from build123d import *

# Parameters (mm, degrees)
SKETCH1_W           = 138
SKETCH1_H           = 108.5
SKETCH1_R           = 1.75
BOSS_EXTRUDE1_DEPTH = 10


with BuildPart() as part:
    # Sketch1 → Boss-Extrude1 (new body)
    with BuildSketch(Plane(origin=(0, 0, 0), x_dir=(1, 0, 0), z_dir=(0, 1, 0))):
        Rectangle(SKETCH1_W, SKETCH1_H)
        with Locations(Location((-64, 49, 0), (0, 0, 270))):  # turned: the seam where the file's is
            Circle(SKETCH1_R, mode=Mode.SUBTRACT)
        with Locations(Location((-64, -49, 0), (0, 0, 270))):  # turned: the seam where the file's is
            Circle(SKETCH1_R, mode=Mode.SUBTRACT)
        with Locations(Location((64, -49, 0), (0, 0, 270))):  # turned: the seam where the file's is
            Circle(SKETCH1_R, mode=Mode.SUBTRACT)
        with Locations(Location((64, 49, 0), (0, 0, 270))):  # turned: the seam where the file's is
            Circle(SKETCH1_R, mode=Mode.SUBTRACT)
        with Locations(Location((-57.5, 44, 0), (0, 0, 270))):  # turned: the seam where the file's is
            Circle(SKETCH1_R, mode=Mode.SUBTRACT)
        with Locations(Location((-17.5, 44, 0), (0, 0, 270))):  # turned: the seam where the file's is
            Circle(SKETCH1_R, mode=Mode.SUBTRACT)
        with Locations(Location((-17.5, -44, 0), (0, 0, 270))):  # turned: the seam where the file's is
            Circle(SKETCH1_R, mode=Mode.SUBTRACT)
        with Locations(Location((-57.5, -44, 0), (0, 0, 270))):  # turned: the seam where the file's is
            Circle(SKETCH1_R, mode=Mode.SUBTRACT)
        with Locations(Location((17.5, -44, 0), (0, 0, 270))):  # turned: the seam where the file's is
            Circle(SKETCH1_R, mode=Mode.SUBTRACT)
        with Locations(Location((57.5, -44, 0), (0, 0, 270))):  # turned: the seam where the file's is
            Circle(SKETCH1_R, mode=Mode.SUBTRACT)
        with Locations(Location((57.5, 44, 0), (0, 0, 270))):  # turned: the seam where the file's is
            Circle(SKETCH1_R, mode=Mode.SUBTRACT)
        with Locations(Location((17.5, 44, 0), (0, 0, 270))):  # turned: the seam where the file's is
            Circle(SKETCH1_R, mode=Mode.SUBTRACT)
    extrude(amount=BOSS_EXTRUDE1_DEPTH)


solid = part.part
The listing builds one solid part. Answer for the finished solid, in the listing's coordinates (mm). Give positions to 0.01 mm unless a question says otherwise; leave off trailing zeros. Write each loop counter-clockwise with the first axis right and the second up, starting at its lowest first coordinate (ties: lowest second). Pieces come first, ordered by that corner, then holes. Notation, with made-up numbers: (8.5, -33) -> (60.5, -33) arc R26 cw to (60.5, -3) -> close; hole circle Ø10 at (59.25, 62.25). An arc over 180 degrees is marked (long way). One line per question, with ' | ' between items. Start each with the question number.
1. Section B-B (x = -57.5) is taken. Determine the outline of the cut face in (y, z).
2. Section A-A (z = -49) is taken. Determine the outline of the cut face in (x, y), plus the area to 3 significant figures.
3. Given pin 1 Ø3 at (x, z) = (-64, -49) entering from +Y, flat-ended and moving along its own axis, determine where the tip first touches the part or whether it passes through.
4. For a pull along X with two mould halves and no side action, classify faces 1 (the cylindrical face through (56.83, 4.93, 45.617)), 2 (the cylindrical face through (-16.974, 4.93, 45.669)), 3 (the flat face through (-1, 0, -1)), 4 (the flat face through (-69, 5, 1)) as pulls with the +X half, pulls with the -X half, needs draft (parallel to the pull), parting line crosses it, or undercut.
5. Find the intervals of material crossed by probe 1 along X at (y, z) = (4.25, -44); probe 2 along X at (y, z) = (6.5, -49); probe 3 along Z at (x, y) = (64, 5.5), in increasing order.
Response values:
1) outline: (0, -54.25) -> (10, -54.25) -> (10, -45.75) -> (0, -45.75) -> close; (0, -42.25) -> (10, -42.25) -> (10, 42.25) -> (0, 42.25) -> close; (0, 45.75) -> (10, 45.75) -> (10, 54.25) -> (0, 54.25) -> close
2) outline: (-69, 0) -> (-65.75, 0) -> (-65.75, 10) -> (-69, 10) -> close; (-62.25, 0) -> (62.25, 0) -> (62.25, 10) -> (-62.25, 10) -> close; (65.75, 0) -> (69, 0) -> (69, 10) -> (65.75, 10) -> close | area: 1,310 mm2
3) pin 1: through
4) face 1: undercut | face 2: undercut | face 3: needs draft | face 4: pulls with the -X half
5) probe 1: -69 to -59.25, -55.75 to -19.25, -15.75 to 15.75, 19.25 to 55.75, 59.25 to 69 | probe 2: -69 to -65.75, -62.25 to 62.25, 65.75 to 69 | probe 3: -54.25 to -50.75, -47.25 to 47.25, 50.75 to 54.25
